Read the model definition and answer for the solid it produces. Units are mm, in the model's axes. Round coordinates to 2 decimals unless told otherwise and drop trailing zeros. Loops run counter-clockwise (first coordinate to the right, second up) from the corner with the lowest first, then second, coordinate; pieces in that order, holes last. Notation, with made-up numbers: M 48,6 L 83,6 A20 cw 83,21 Z; hole C 85.25,-39.5 d8. An arc over 180 degrees is marked long. Answer as CSV lines item,"result".
```python
from build123d import *

# Parameters (mm, degrees)
SKETCH1_R           = 9
BOSS_EXTRUDE1_DEPTH = 1.5
SKETCH2_R           = 5
BOSS_EXTRUDE2_DEPTH = 1
SKETCH3_R           = 9
BOSS_EXTRUDE3_DEPTH = 1.5
SKETCH4_R           = 1
CUT_EXTRUDE1_DEPTH  = 14.341664064
BOSS_EXTRUDE4_START = -4
SKETCH6_R           = 1
BOSS_EXTRUDE4_DEPTH = 4


with BuildPart() as part:
    # Sketch1 → Boss-Extrude1 (new body)
    with BuildSketch(Plane(origin=(0, 0, 0), x_dir=(1, 0, 0), z_dir=(0, 1, 0))):
        with Locations(Location((0, 0, 0), (0, 0, 270))):
            Circle(SKETCH1_R)
    extrude(amount=BOSS_EXTRUDE1_DEPTH)

    # Sketch2 → Boss-Extrude2 (add)
    with BuildSketch(Plane(origin=(0, 1.5, 0), x_dir=(1, 0, 0), z_dir=(0, 1, 0))):
        with Locations(Location((0, 0, 0), (0, 0, 270))):
            Circle(SKETCH2_R)
    extrude(amount=BOSS_EXTRUDE2_DEPTH)

    # Sketch3 → Boss-Extrude3 (add)
    with BuildSketch(Plane(origin=(0, 2.5, 0), x_dir=(1, 0, 0), z_dir=(0, 1, 0))):
        with Locations(Location((0, 0, 0), (0, 0, 270))):
            Circle(SKETCH3_R)
    extrude(amount=BOSS_EXTRUDE3_DEPTH)

    # Sketch4 → Cut-Extrude1 (cut, through all)
    with BuildSketch(Plane.XZ):
        with Locations(Location((0, 7, 0), (0, 0, 270))):
            Circle(SKETCH4_R)
        with Locations(Location((3.5, 6.062177826, 0), (0, 0, 270))):
            Circle(SKETCH4_R)
        with Locations(Location((6.062177826, 3.5, 0), (0, 0, 270))):
            Circle(SKETCH4_R)
        with Locations(Location((7, 0, 0), (0, 0, 270))):
            Circle(SKETCH4_R)
        with Locations(Location((6.062177826, -3.5, 0), (0, 0, 270))):
            Circle(SKETCH4_R)
        with Locations(Location((3.5, -6.062177826, 0), (0, 0, 270))):
            Circle(SKETCH4_R)
        with Locations(Location((0, -7, 0), (0, 0, 270))):
            Circle(SKETCH4_R)
        with Locations(Location((-3.5, -6.062177826, 0), (0, 0, 270))):
            Circle(SKETCH4_R)
        with Locations(Location((-6.062177826, -3.5, 0), (0, 0, 270))):
            Circle(SKETCH4_R)
        with Locations(Location((-7, 0, 0), (0, 0, 270))):
            Circle(SKETCH4_R)
        with Locations(Location((-6.062177826, 3.5, 0), (0, 0, 270))):
            Circle(SKETCH4_R)
        with Locations(Location((-3.5, 6.062177826, 0), (0, 0, 270))):
            Circle(SKETCH4_R)
    extrude(amount=-CUT_EXTRUDE1_DEPTH, mode=Mode.SUBTRACT)

    # Sketch6 → Boss-Extrude4 (add)
    with BuildSketch(Plane(origin=(0, 4, 0), x_dir=(1, 0, 0), z_dir=(0, 1, 0)).offset(BOSS_EXTRUDE4_START)):
        with Locations(Location((-3.5, -6.062177826, 0), (0, 0, 270))):
            Circle(SKETCH6_R)
    extrude(amount=BOSS_EXTRUDE4_DEPTH)


solid = part.part
```
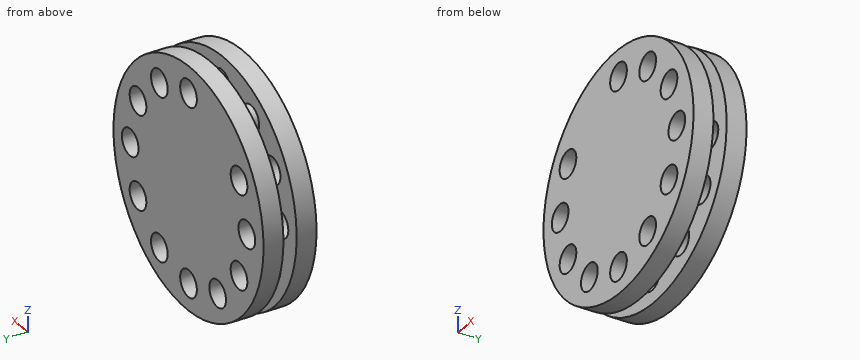
1) Each of these flat-tipped pins is pushed along its axis until it touches: P1, Ø1.8, axis at x = 3.5, z = -6.06, coming from the -Y side; P2, Ø1.5, axis at y = 1.5, z = 5, coming from the -X side; P3, Ø1.5, axis at x = 6, y = 1, coming from the +Z side. Where does it stop, or does it pass through?
Evaluation:
P1,"passes through"
P2,"stops at x = -7.93"
P3,"stops at z = 7.31"
2) Find section B-B, the plane z = -7.5. Give the vertices of the cut face in (x, y).
Evaluation:
outline,"M -4.97,0 L -0.87,0 L -0.87,1.5 L -4.97,1.5 Z; M -4.97,2.5 L -0.87,2.5 L -0.87,4 L -4.97,4 Z; M 0.87,0 L 4.97,0 L 4.97,1.5 L 0.87,1.5 Z; M 0.87,2.5 L 4.97,2.5 L 4.97,4 L 0.87,4 Z"
3) Find section C-C, the plane x = 3.5. Give the vertices of the cut face in (y, z).
Evaluation:
outline,"M 0,-8.29 L 1.5,-8.29 L 1.5,-7.06 L 0,-7.06 Z; M 0,-5.06 L 1.5,-5.06 L 1.5,-3.57 L 2.5,-3.57 L 2.5,-5.06 L 4,-5.06 L 4,5.06 L 2.5,5.06 L 2.5,3.57 L 1.5,3.57 L 1.5,5.06 L 0,5.06 Z; M 0,7.06 L 1.5,7.06 L 1.5,8.29 L 0,8.29 Z; M 2.5,-8.29 L 4,-8.29 L 4,-7.06 L 2.5,-7.06 Z; M 2.5,7.06 L 4,7.06 L 4,8.29 L 2.5,8.29 Z"
4) Find section D-D, the plane z = -3.5. Give the vertices of the cut face in (x, y).
Evaluation:
outline,"M -8.29,0 L -7.06,0 L -7.06,1.5 L -8.29,1.5 Z; M -8.29,2.5 L -7.06,2.5 L -7.06,4 L -8.29,4 Z; M -5.06,0 L 5.06,0 L 5.06,1.5 L 3.57,1.5 L 3.57,2.5 L 5.06,2.5 L 5.06,4 L -5.06,4 L -5.06,2.5 L -3.57,2.5 L -3.57,1.5 L -5.06,1.5 Z; M 7.06,0 L 8.29,0 L 8.29,1.5 L 7.06,1.5 Z; M 7.06,2.5 L 8.29,2.5 L 8.29,4 L 7.06,4 Z"
5) Straight lines are drawn through the part: line 1 (X direction, y = 3.35, z = 0); line 2 (Z direction, x = 4, y = 3.65); line 3 (X direction, y = 0.9, z = -3.5). For each, find the intervals that lie inside material, in ascending order.
Evaluation:
line 1,"x = -9 to -8, -6 to 6, 8 to 9"
line 2,"z = -8.06 to -6.93, -5.2 to 5.2, 6.93 to 8.06"
line 3,"x = -8.29 to -7.06, -5.06 to 5.06, 7.06 to 8.29"
6) Find section A-A, the plane x = -3.5. Give the vertices of the cut face in (y, z).
Evaluation:
outline,"M 0,-8.29 L 1.5,-8.29 L 1.5,-7.06 L 0,-7.06 Z; M 0,-5.06 L 1.5,-5.06 L 1.5,-3.57 L 2.5,-3.57 L 2.5,-5.06 L 4,-5.06 L 4,8.29 L 2.5,8.29 L 2.5,7.06 L 1.5,7.06 L 1.5,8.29 L 0,8.29 Z; M 2.5,-8.29 L 4,-8.29 L 4,-7.06 L 2.5,-7.06 Z; hole M 1.5,3.57 L 2.5,3.57 L 2.5,5.06 L 1.5,5.06 Z"
